Work out the finished part from the listing and answer in its coordinate system (mm). Face numbers are marked on the shaded views. Coordinates: 2 decimals unless noted, no trailing zeros. Loops run counter-clockwise (first coordinate to the right, second up) from the corner with the lowest first, then second, coordinate; pieces in that order, holes last. Notation, with made-up numbers: (54.5, 54.25) -> (74.5, 54.25) arc R9 cw to (74.5, 62.25) -> close; hole circle Ø8 at (57.25, 46). An arc over 180 degrees is marked (long way). Use a Markdown table: item, result.
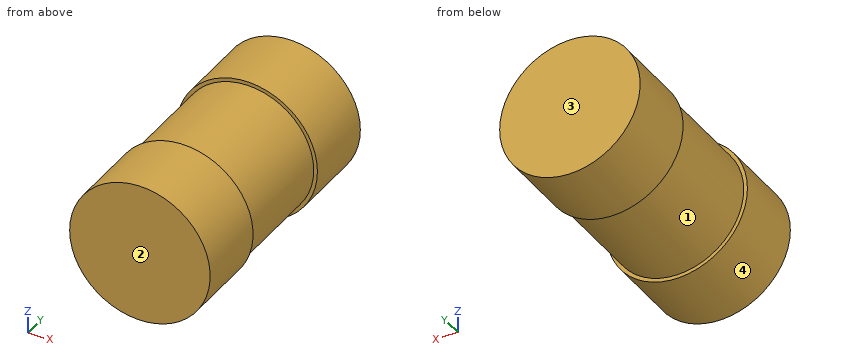
from build123d import *

# Parameters (mm, degrees)
SKETCH1_R           = 9
BOSS_EXTRUDE1_DEPTH = 35
SKETCH2_R           = 9.5
SKETCH2_R_2         = 9
BOSS_EXTRUDE2_DEPTH = 10
SKETCH3_R           = 9.5
SKETCH3_R_2         = 9
BOSS_EXTRUDE3_DEPTH = 10


with BuildPart() as part:
    # Sketch1 → Boss-Extrude1 (new body)
    with BuildSketch(Plane(origin=(0, 0, 0), x_dir=(1, 0, 0), z_dir=(0, 1, 0))):
        Circle(SKETCH1_R)
    extrude(amount=BOSS_EXTRUDE1_DEPTH)

    # Sketch2 → Boss-Extrude2 (add)
    with BuildSketch(Plane(origin=(0, 35, 0), x_dir=(1, 0, 0), z_dir=(0, 1, 0))):
        Circle(SKETCH2_R)
        Circle(SKETCH2_R_2, mode=Mode.SUBTRACT)
    extrude(amount=-BOSS_EXTRUDE2_DEPTH)

    # Sketch3 → Boss-Extrude3 (add)
    with BuildSketch(Plane(origin=(0, 0, 0), x_dir=(-1, 0, 0), z_dir=(0, -1, 0))):
        Circle(SKETCH3_R)
        Circle(SKETCH3_R_2, mode=Mode.SUBTRACT)
    extrude(amount=-BOSS_EXTRUDE3_DEPTH)


solid = part.part
Q1. Consider line 1 (Y direction, x = -8, z = 5); line 2 (X direction, y = 19, z = -0.25); line 3 (Z direction, x = -1.5, y = 8.5). Determine where each line is inside the solid, lowest interval first. Write a range as [from, to].
Solved:
| item | result |
|---|---|
| line 1 | [0, 10], [25, 35] |
| line 2 | [-9, 9] |
| line 3 | [-9.38, 9.38] |
Q2. Section B-B on x = 0 is taken. Determine the outline of the cut face in (y, z), and give its area (3 significant figures).
Solved:
| item | result |
|---|---|
| outline | (0, -9.5) -> (10, -9.5) -> (10, -9) -> (25, -9) -> (25, -9.5) -> (35, -9.5) -> (35, 9.5) -> (25, 9.5) -> (25, 9) -> (10, 9) -> (10, 9.5) -> (0, 9.5) -> close |
| area | 650 mm² |
Q3. Determine the mould class of the marked faces 1, 2, 3 and 4 for opening direction Y: pulls with the +Y half, pulls with the -Y half, needs draft (parallel to the pull), parting line crosses it, or undercut.
Solved:
| item | result |
|---|---|
| face 1 | undercut |
| face 2 | pulls with the -Y half |
| face 3 | pulls with the +Y half |
| face 4 | needs draft |
Q4. Section D-D on y = 4.5 is taken. Determine the outline of the cut face in (x, z), and give its area (3 significant figures).
Solved:
| item | result |
|---|---|
| outline | circle Ø19 at (0, 0) |
| area | 284 mm² |
Q5. Section C-C on y = 23.5 is taken. Determine the outline of the cut face in (x, z).
Solved:
| item | result |
|---|---|
| outline | circle Ø18 at (0, 0) |
Q6. Section A-A on z = 0 is taken. Determine the outline of the cut face in (x, y), and give its area (3 significant figures).
Solved:
| item | result |
|---|---|
| outline | (-9.5, 0) -> (9.5, 0) -> (9.5, 10) -> (9, 10) -> (9, 25) -> (9.5, 25) -> (9.5, 35) -> (-9.5, 35) -> (-9.5, 25) -> (-9, 25) -> (-9, 10) -> (-9.5, 10) -> close |
| area | 650 mm² |
Q7. Given pin 1 Ø1 at (y, z) = (6.5, 3.5) entering from +X, flat-ended and moving along its own axis, determine where the tip first touches the part or whether it passes through.
Solved:
| item | result |
|---|---|
| pin 1 | x = 9.01 |
